Autodesk Inventor part; units mm, degrees
ref_plane "YZ Plane" through (0, 0, 0) normal (1, 0, 0) x (0, 1, 0)
ref_plane "XZ Plane" through (0, 0, 0) normal (0, 1, 0) x (-1, 0, 0)
ref_plane "XY Plane" through (0, 0, 0) normal (0, 0, 1) x (1, 0, 0)
sketch "Sketch1" plane through (0, 0, 0) normal (0, 1, 0) x (-1, 0, 0)
  line L0 (0, 0) -> (47.625, 0)
  line L1 (47.625, 0) -> (47.625, -22.225)
  line L2 (47.625, -22.225) -> (0, -22.225)
  line L3 (0, -22.225) -> (0, 0)
  dimension "d0" = 22.225
  dimension "d1" = 47.625
extrude "Extrusion1" add sketch "Sketch1" along normal blind 1.27
sketch "Sketch2" plane through (0, 1.27, 0) normal (0, 1, 0) x (1, 0, 0)
  circle A0 centre (-6.985, 3.4925) radius 0.762
  line L0 (-47.625, 0) -> (0, 0) construction
  line L1 (0, 0) -> (0, 22.225) construction
  line L2 (0, 22.225) -> (-47.625, 22.225) construction
  line L3 (-47.625, 22.225) -> (-47.625, 0) construction
  circle A1 centre (-9.525, 3.4925) radius 0.762
  circle A2 centre (-12.065, 3.4925) radius 0.762
  circle A3 centre (-14.605, 3.4925) radius 0.762
  circle A4 centre (-17.145, 3.4925) radius 0.762
  circle A5 centre (-19.685, 3.4925) radius 0.762
  circle A6 centre (-22.225, 3.4925) radius 0.762
  circle A7 centre (-24.765, 3.4925) radius 0.762
  circle A8 centre (-27.305, 3.4925) radius 0.762
  circle A9 centre (-29.845, 3.4925) radius 0.762
  circle A10 centre (-32.385, 3.4925) radius 0.762
  circle A11 centre (-34.925, 3.4925) radius 0.762
  circle A12 centre (-37.465, 3.4925) radius 0.762
  circle A13 centre (-40.005, 3.4925) radius 0.762
  circle A14 centre (-42.545, 3.4925) radius 0.762
  circle A15 centre (-6.985, 18.7325) radius 0.762
  circle A16 centre (-9.525, 18.7325) radius 0.762
  circle A17 centre (-12.065, 18.7325) radius 0.762
  circle A18 centre (-14.605, 18.7325) radius 0.762
  circle A19 centre (-17.145, 18.7325) radius 0.762
  circle A20 centre (-19.685, 18.7325) radius 0.762
  circle A21 centre (-22.225, 18.7325) radius 0.762
  circle A22 centre (-24.765, 18.7325) radius 0.762
  circle A23 centre (-27.305, 18.7325) radius 0.762
  circle A24 centre (-29.845, 18.7325) radius 0.762
  circle A25 centre (-32.385, 18.7325) radius 0.762
  circle A26 centre (-34.925, 18.7325) radius 0.762
  circle A27 centre (-37.465, 18.7325) radius 0.762
  circle A28 centre (-40.005, 18.7325) radius 0.762
  circle A29 centre (-42.545, 18.7325) radius 0.762
  dimension "d4" = 1.524
  dimension "d5" = 3.4925
  dimension "d6" = 6.985
  dimension "d9" = 2.54
  dimension "d12" = 15.24
extrude "Extrusion2" cut sketch "Sketch2" against normal through all
fillet "Fillet1" radius 1.27 4 edges at (-47.625, 0.635, 0) (-47.625, 0.635, -22.225) (0, 0.635, 0) (0, 0.635, -22.225)
properties part number "BackupNanoCasePart2" material "ABS Plastic"
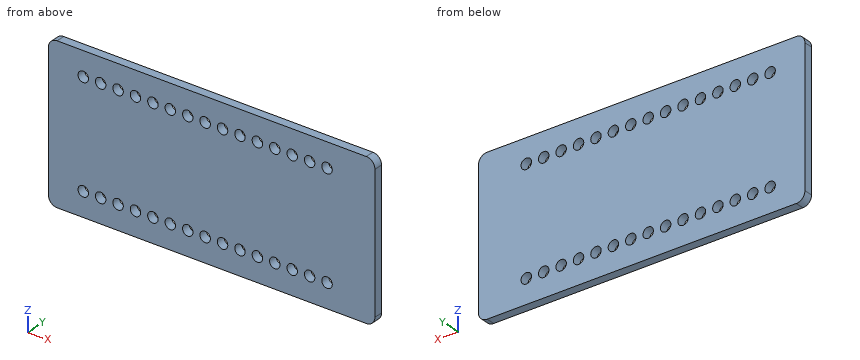
Input: part model. Units: mm. Frame: model coordinates. Coordinates: 2 decimals unless noted, no trailing zeros. Loops run counter-clockwise (first coordinate to the right, second up) from the corner with the lowest first, then second, coordinate; pieces in that order, holes last.
Q1. Section B-B, the plane y = 0.45. Give the number of separate pieces and of enclosed holes in the cut face, and give its area (3 significant figures).
Results are:
separate pieces: 1
enclosed holes: 30
area: 1,000 mm2
Q2. Section A-A, the plane x = -12. Return the cut outline in (y, z) (3 decimals), and give its area (3 significant figures).
Results are:
outline: (0, -22.225) - (1.27, -22.225) - (1.27, -19.492) - (0, -19.492) - close; (0, -17.973) - (1.27, -17.973) - (1.27, -4.252) - (0, -4.252) - close; (0, -2.733) - (1.27, -2.733) - (1.27, 0) - (0, 0) - close
area: 24.4 mm2
Q3. Contact query for a flat-ended pin moving along its axis: pin 1 (0.9 mm diameter, centred on x = -24.76, z = -18.73, fed in from -Y). Output: stop coordinate, or through.
Results are:
pin 1: passes through
Q4. Line query: line 1 along Z through (x, y) = (-37.5, 0.3) (3 decimals); line 2 along Z through (x, y) = (-11.5, 0.2) (3 decimals). Output: solid intervals per line, ascending.
Results are:
line 1: z = -22.225 to -19.494, -17.971 to -4.254, -2.731 to 0
line 2: z = -22.225 to -19.244, -18.221 to -4.004, -2.981 to 0
